Work out the finished part from the listing and answer in its coordinate system (mm). A direction names the side the tool comes from. Coordinates: 2 decimals unless noted, no trailing zeros. Write each loop counter-clockwise with the first axis right and the second up, starting at its lowest first coordinate (ties: lowest second). Pieces come first, ordered by that corner, then holes. Notation, with made-up numbers: (31, 74.25) - (49, 74.25) arc R20 ccw to (49, 102.25) - close; hole circle Ø5 at (82, 45). An arc over 180 degrees is marked (long way). Use a Markdown table: item, result. Add a question column.
(1) The part is cut by section D-D, the plane x = -57.5. Give the vertices of the cut face in (y, z), then the cut area to 3 significant figures.
(2) Find the intervals of material crossed by line 1 (Z direction, x = -54.75, y = 4.5); line 2 (Z direction, x = -35, y = 7.75); line 3 (Y direction, x = -37.75, z = 113.5), in increasing order. Write a range as from..to.
(3) A tool of negligible diameter and unlimited length cuts with its end or side. For faces 1 (the face through (-39, 0, 218)), 2 (the face through (-52, 15, 207)), 3 (the face through (-46, 25, 139)), 4 (the face through (-52, 15, 73.331)), from which of +Z, -Z, +X, -X, +Y, -Y can it reach the whole face along a straight path? Write none if from no direction.
(4) The part is cut by section C-C, the plane z = 69.5. Give the vertices of the cut face in (x, y).
(5) The part is cut by section A-A, the plane y = 12. Give the vertices of the cut face in (x, z).
(6) Given pin 1 Ø10 at (x, z) = (-52, 145.5) entering from -Y; pin 2 Ø8 at (y, z) = (8.5, 224.5) entering from -X; pin 3 Ø10 at (x, y) = (-52, 12) entering from +Z; pin 4 Ø6 at (x, z) = (-48.5, 64.5) entering from +Y, each flat-ended and moving along its own axis, determine where each tip first touches the part or whether it passes through.
(7) For a pull along Z with two mould halves and no side action, classify faces 5 (the face through (-38, 15, 44.5)), 6 (the face through (-45, 12, 201.5)), 7 (the face through (-38, 15, 234.5)), 8 (the face through (-31.29, 28, 138)) as released by +Z, released by -Z, zero draft, split by the parting line, or undercut.
(8) The part is cut by section B-B, the plane x = -33.5. Give the vertices of the cut face in (y, z), then the cut area to 3 significant figures.
Autodesk Inventor part; units mm, degrees
ref_plane "YZ Plane" through (0, 0, 0) normal (1, 0, 0) x (0, 1, 0)
ref_plane "XZ Plane" through (0, 0, 0) normal (0, 1, 0) x (-1, 0, 0)
ref_plane "XY Plane" through (0, 0, 0) normal (0, 0, 1) x (1, 0, 0)
sketch "Эскиз1" plane through (0, 0, 0) normal (0, 1, 0) x (-1, 0, 0)
  line L0 (44.4709, 73.3307) -> (60, 73.3307)
  line L1 (44.4709, 73.3307) -> (44.4709, 28.3307)
  line L2 (44.4709, 207.0004) -> (60, 207.0004)
  line L3 (44.4709, 207.0004) -> (44.4709, 252.0004)
  line L4 (31.29, 29.5004) -> (31.29, 249.5004)
  line L5 (31.29, 201.5002) -> (60, 201.5002)
  line L6 (60, 78.8309) -> (31.29, 78.8309)
  line L7 (44.4709, 234.5004) -> (31.29, 234.5004)
  line L8 (44.4709, 44.5004) -> (31.29, 44.5004)
  line L9 (31.29, 139.5004) -> (37.8804, 139.5004)
  line L10 (60, 207.0004) -> (60, 201.5002)
  line L11 (60, 78.8309) -> (60, 73.3307)
  point P0 (0, 0)
  dimension "d0" = 5.5002
  dimension "d1" = 5.5002
  dimension "d2" = 95
extrude "Выдавливание1" add sketch "Эскиз1" along normal blind 30
sketch "Эскиз2" plane through (0, 30, 0) normal (0, 1, 0) x (1, 0, 0)
  line L0 (-60, -201.5002) -> (-60, -207.0004)
  line L1 (-31.29, -78.8309) -> (-31.29, -44.5004)
  line L2 (-60, -207.0004) -> (-31.29, -207.0004)
  line L3 (-31.29, -207.0004) -> (-31.29, -73.3307)
  line L4 (-31.29, -73.3307) -> (-60, -73.3307)
  line L5 (-60, -73.3307) -> (-60, -207.0004)
  point P0 (0, 0)
extrude "Выдавливание2" add sketch "Эскиз2" against normal blind 5
equation "\"d1\" = d0"
properties part number "KB33-046-010 - Панель управления"
Model answer:
| question | item | result |
|---|---|---|
| 1 | outline | (0, 73.33) - (30, 73.33) - (30, 207) - (0, 207) - (0, 201.5) - (25, 201.5) - (25, 78.83) - (0, 78.83) - close |
| 1 | area | 943 mm^2 |
| 2 | line 1 | 73.33..78.83, 201.5..207 |
| 2 | line 2 | 44.5..78.83, 201.5..234.5 |
| 2 | line 3 | 25..30 |
| 3 | face 1 | +Z, -Z, +X, -X, -Y |
| 3 | face 2 | +Z, -X, +Y, -Y |
| 3 | face 3 | +X, -X, -Y |
| 3 | face 4 | -Z, -X, +Y, -Y |
| 4 | outline | (-44.47, 0) - (-31.29, 0) - (-31.29, 30) - (-44.47, 30) - close |
| 5 | outline | (-60, 73.33) - (-44.47, 73.33) - (-44.47, 44.5) - (-31.29, 44.5) - (-31.29, 78.83) - (-60, 78.83) - close; (-60, 201.5) - (-31.29, 201.5) - (-31.29, 234.5) - (-44.47, 234.5) - (-44.47, 207) - (-60, 207) - close |
| 6 | pin 1 | y = 25 |
| 6 | pin 2 | x = -44.47 |
| 6 | pin 3 | z = 207 |
| 6 | pin 4 | through |
| 7 | face 5 | released by -Z |
| 7 | face 6 | undercut |
| 7 | face 7 | released by +Z |
| 7 | face 8 | zero draft |
| 8 | outline | (0, 44.5) - (30, 44.5) - (30, 234.5) - (0, 234.5) - (0, 201.5) - (25, 201.5) - (25, 78.83) - (0, 78.83) - close |
| 8 | area | 2,630 mm^2 |
